Design review of the part built by this model. Coordinates are the model's own, in mm. A direction names the side the tool comes from. Coordinates: 2 decimals unless noted, no trailing zeros. Loops run counter-clockwise (first coordinate to the right, second up) from the corner with the lowest first, then second, coordinate; pieces in that order, holes last.
from build123d import *

# Parameters (mm, degrees)
F0_R          = 19.05
F1_DEPTH      = 31.75
F2_DEPTH      = 4.7625
F3_R          = 5.5626
F4_DEPTH      = 15.875
F4_DEPTH_BACK = 4.7752
F5_DEPTH      = 63.501


with BuildPart() as f1:
    # F0 (on Front) → F1 (new body, symmetric)
    with BuildSketch(Plane.XZ):
        with BuildLine():
            Line((50.8, 31.75), (0, 31.75))
            ThreePointArc((0, 31.75), (-29.9181979044, -10.6284492827), (20.0304912791, -24.6341616281))
            ThreePointArc((20.0304912791, -24.6341616281), (29.6377097996, -11.3872146654), (31.3720103364, 4.8846153846))
            ThreePointArc((31.3720103364, 4.8846153846), (33.5488565837, 12.545475629), (40.7836134373, 15.875))
            Line((40.7836134373, 15.875), (50.8, 15.875))
            Line((50.8, 15.875), (50.8, 31.75))
        make_face()
        Circle(F0_R, mode=Mode.SUBTRACT)
    extrude(amount=F1_DEPTH, both=True)

    # F0 (on Front) → F2 (join, symmetric)
    with BuildSketch(Plane.XZ):
        with BuildLine():
            ThreePointArc((31.3720103364, 4.8846153846), (29.6377097996, -11.3872146654), (20.0304912791, -24.6341616281))
            Line((20.0304912791, -24.6341616281), (69.85, 15.875))
            Line((69.85, 15.875), (50.8, 15.875))
            Line((50.8, 15.875), (40.7836134373, 15.875))
            ThreePointArc((40.7836134373, 15.875), (33.5488565837, 12.545475629), (31.3720103364, 4.8846153846))
        make_face()
    extrude(amount=F2_DEPTH, both=True)

    # F3 (on face) → F4 (join, two sides)
    with BuildSketch(Plane.XY.offset(31.75)) as f4_sk:
        with BuildLine():
            ThreePointArc((57.0991554441, 30.0777214642), (54.0586759125, 31.3248128824), (50.8, 31.75))
            Line((50.8, 31.75), (50.8, 24.6126))
            ThreePointArc((50.8, 24.6126), (54.733352181, 22.983352181), (56.3626, 19.05))
            ThreePointArc((56.3626, 19.05), (54.733352181, 15.116647819), (50.8, 13.4874))
            Line((50.8, 13.4874), (50.8, -13.4874))
            ThreePointArc((50.8, -13.4874), (54.733352181, -15.116647819), (56.3626, -19.05))
            ThreePointArc((56.3626, -19.05), (54.733352181, -22.983352181), (50.8, -24.6126))
            Line((50.8, -24.6126), (50.8, -31.75))
            ThreePointArc((50.8, -31.75), (54.0586759125, -31.3248128824), (57.0991554441, -30.0777214642))
            Line((57.0991554441, -30.0777214642), (90.4493554441, -11.0277214642))
            ThreePointArc((90.4493554441, -11.0277214642), (96.8502, 0), (90.4493554441, 11.0277214642))
            Line((90.4493554441, 11.0277214642), (57.0991554441, 30.0777214642))
        make_face()
        with Locations((84.1502, 0)):
            Circle(F3_R, mode=Mode.SUBTRACT)
        with BuildLine():
            Line((50.8, 24.6126), (50.8, 31.75))
            ThreePointArc((50.8, 31.75), (41.8197438789, 28.0302561211), (38.1, 19.05))
            Line((38.1, 19.05), (38.1, -19.05))
            ThreePointArc((38.1, -19.05), (41.8197438789, -28.0302561211), (50.8, -31.75))
            Line((50.8, -31.75), (50.8, -24.6126))
            ThreePointArc((50.8, -24.6126), (45.2374, -19.05), (50.8, -13.4874))
            Line((50.8, -13.4874), (50.8, 13.4874))
            ThreePointArc((50.8, 13.4874), (45.2374, 19.05), (50.8, 24.6126))
        make_face()
    extrude(amount=-F4_DEPTH)
    extrude(f4_sk.sketch, amount=F4_DEPTH_BACK)

    # F5 (cut, through all): faces of the model
    f5_faces = [f1.faces().sort_by_distance(p)[0] for p in [
        (48.4391592362, -19.05, 31.75),
        (48.4391592362, 19.05, 31.75),
    ]]
    extrude(f5_faces, amount=-F5_DEPTH, mode=Mode.SUBTRACT)


solid = f1.part
Q1. Take a section at B-B, the plane z = 0. Write out the cut boundary in (x, y), then the cut area to 3 significant figures.
Q2. Machinability: for faces 5 (the flat face through (62, 8, 15.875)), 6 (the flat face through (38.1, 0, 34)), 7 (the cylindrical face through (33.475, 18.067, 12.458)), 8 (the flat face through (18, -31.75, 8)), 9 (the cylindrical face through (33.475, -18.445, 12.458)), which of the approach directions +Z, -Z, +X, -X, +Y, -Y give a long, thin tool a straight path to every point of the face, cutting with its end or side? Answer none if there is none.
Q3. Take a section at C-C, the plane x = 62.5. Write out the cut boundary in (y, z) (1 decimal), then the cut area to 3 significant figures.
Q4. For line 1 (X direction, y = 7, z = 0.5); line 2 (X direction, y = 20, z = 16); line 3 (Z direction, x = 83, y = -6) (3 decimals), list the stretches that pass through material, from the lowest coordinate up.
Q5. Clearance check with flat-ended pins moving along their axes: pin 1 Ø10 at (x, y) = (84.15, 0) entering from -Z; pin 2 Ø8 at (y, z) = (4.5, 13.5) entering from +X; pin 3 Ø5 at (x, z) = (49, 0.5) entering from +Y; pin 4 Ø2 at (x, y) = (45.5, -7.5) entering from -Z (3 decimals). State where each tip first meets the part, or that it passes through.
Q6. Take a section at A-A, the plane x = -9. Write out the cut boundary in (y, z).
Q7. The part is to be moulded in two halves that separate along X. For faces 1 (the flat face through (61, 0, 36.525)), 2 (the cylindrical face through (-21.46, -0.44, -23.4)), 3 (the flat face through (44.592, -0.067, -4.663)), 4 (the cylindrical face through (78.593, 0.245, 26.056)), say which applies: pulls with the +X half, pulls with the -X half, needs draft (parallel to the pull), parting line crosses it, or undercut.
Q8. Take a section at D-D, the plane z = -22.5. Write out the cut boundary in (x, y), then the cut area to 3 significant figures.
Entries:
1. outline: (-31.75, -31.75) - (-19.05, -31.75) - (-19.05, 31.75) - (-31.75, 31.75) - close; (19.05, -31.75) - (31.75, -31.75) - (31.75, -4.76) - (50.33, -4.76) - (50.33, 4.76) - (31.75, 4.76) - (31.75, 31.75) - (19.05, 31.75) - close
1. area: 1,790 mm2
2. face 5: -Z, +X
2. face 6: +Z, -X, +Y, -Y
2. face 7: +X, +Y
2. face 8: +Z, -Z, +X, -X, -Y
2. face 9: +X, -Y
3. outline: (-27, 15.9) - (-4.8, 15.9) - (-4.8, 9.9) - (4.8, 9.9) - (4.8, 15.9) - (27, 15.9) - (27, 36.5) - (-27, 36.5) - close
3. area: 1,170 mm2
4. line 1: x = -31.75 to -19.04, 19.04 to 31.75
4. line 2: x = -27.42 to -10.34, 10.34 to 45.32, 56.28 to 74.74
4. line 3: z = 15.875 to 36.525
5. pin 1: passes through
5. pin 2: stops at x = 96.79
5. pin 3: stops at y = 4.76
5. pin 4: stops at z = 15.875
6. outline: (-31.75, -30.45) - (31.75, -30.45) - (31.75, -16.79) - (-31.75, -16.79) - close; (-31.75, 16.79) - (31.75, 16.79) - (31.75, 30.45) - (-31.75, 30.45) - close
7. face 1: needs draft
7. face 2: parting line crosses it
7. face 3: pulls with the +X half
7. face 4: undercut
8. outline: (-22.4, -31.75) - (22.4, -31.75) - (22.4, -4.76) - (22.66, -4.76) - (22.66, 4.76) - (22.4, 4.76) - (22.4, 31.75) - (-22.4, 31.75) - close
8. area: 2,850 mm2
